from build123d import *

# Parameters (mm, degrees)
F1_DEPTH = 75
F2_R     = 110


with BuildPart() as f1:
    # F0 (on Front) → F1 (new body)
    with BuildSketch(Plane.XZ):
        Polygon((21.498629, 113.340293), (51.498629, 0), (171.498629, 0), (171.498629, 113.340293), align=None)
    extrude(amount=F1_DEPTH)

    # F2
    f2_edges = [f1.edges().sort_by_distance(p)[0] for p in [
        (171.498629, -37.5, 113.340293),
    ]]
    fillet(f2_edges, radius=F2_R)


solid = f1.part
Model file for the job. Use its own axes, mm. Round coordinates to 2 decimals unless told otherwise and drop trailing zeros. Loops run counter-clockwise (first coordinate to the right, second up) from the corner with the lowest first, then second, coordinate; pieces in that order, holes last.
1. Drop flat-ended pins along their axis: P1, Ø8, axis at y = -8.5, z = 82, coming from the -X side; P2, Ø3, axis at y = -57.5, z = 35.5, coming from the +X side; P3, Ø12, axis at y = -55, z = 76, coming from the +X side. Give the stop position or say it passes through.
Check values:
P1: stops at x = 28.74
P2: stops at x = 167.14
P3: stops at x = 149
2. Wall check: probe 1 along X at (y, z) = (-11, 66.5); probe 2 along X at (y, z) = (-71, 100.5); probe 3 along Z at (x, y) = (110.5, -65). Give the ranges that are in metal, low to high.
Check values:
probe 1: x = 33.9 to 151.56
probe 2: x = 24.9 to 113.07
probe 3: z = 0 to 101.82
3. Band-saw the part on A-A, the plane y = -50. List the corners of the cut face in (x, z).
Check values:
outline: (21.5, 113.34) - (51.5, 0) - (171.5, 0) - (171.5, 3.34) arc R110 ccw to (61.5, 113.34) - close
4. Band-saw the part on C-C, the plane x = 46. List the corners of the cut face in (y, z).
Check values:
outline: (-75, 20.77) - (0, 20.77) - (0, 113.34) - (-75, 113.34) - close
5. Band-saw the part on B-B, the plane z = 73.5. List the corners of the cut face in (x, y), and give its area (3 significant figures).
Check values:
outline: (32.04, -75) - (146.22, -75) - (146.22, 0) - (32.04, 0) - close
area: 8,560 mm2
